from build123d import *

# Parameters (mm, degrees)
SKETCH1_W           = 41.35
SKETCH1_H           = 35
BOSS_EXTRUDE1_DEPTH = 3.175
SKETCH2_W           = 28.65
SKETCH2_H           = 7.5
SKETCH2_W_2         = 13.075
SKETCH2_H_2         = 3.175
SKETCH2_W_3         = 14.9
CUT_EXTRUDE1_DEPTH  = 4.175


with BuildPart() as part:
    # Sketch1 → Boss-Extrude1 (new body)
    with BuildSketch(Plane(origin=(0, 0, 0), x_dir=(1, 0, 0), z_dir=(0, 1, 0))):
        with Locations((20.675, 17.5)):
            Rectangle(SKETCH1_W, SKETCH1_H)
    extrude(amount=BOSS_EXTRUDE1_DEPTH)

    # Sketch2 → Cut-Extrude1 (cut, through all)
    with BuildSketch(Plane(origin=(0, 3.175, 0), x_dir=(1, 0, 0), z_dir=(0, 1, 0))):
        with Locations((20.675, 23.75)):
            Rectangle(SKETCH2_W, SKETCH2_H)
        with Locations((6.5375, 33.4125)):
            Rectangle(SKETCH2_W_2, SKETCH2_H_2)
        with Locations((34.8125, 33.4125)):
            Rectangle(SKETCH2_W_2, SKETCH2_H_2)
        Polygon((38.175, 21.825), (41.35, 21.825), (41.35, 11.15), (28.275, 11.15), (28.275, 14.325), (38.175, 14.325), align=None)
        Polygon((3.175, 21.825), (3.175, 14.325), (13.075, 14.325), (13.075, 11.15), (0, 11.15), (0, 21.825), align=None)
        with Locations((33.9, 1.5875)):
            Rectangle(SKETCH2_W_3, SKETCH2_H_2)
        with Locations((7.45, 1.5875)):
            Rectangle(SKETCH2_W_3, SKETCH2_H_2)
    extrude(amount=-CUT_EXTRUDE1_DEPTH, mode=Mode.SUBTRACT)


solid = part.part
Source: CAD feature listing. Evaluate the final solid. Frame: model axes, mm. A direction names the side the tool comes from. Round coordinates to 2 decimals unless told otherwise and drop trailing zeros. Loops run counter-clockwise (first coordinate to the right, second up) from the corner with the lowest first, then second, coordinate; pieces in that order, holes last.
Q1. First-contact query: P1, Ø1, axis at x = 40.5, y = 2.5, coming from the +Z side (3 decimals); P2, Ø1, axis at y = 1.5, z = -1.5, coming from the -X side; P3, Ø1, axis at y = 2, z = -33, coming from the -X side (3 decimals). Flat tips, straight axial feed; report the tip coordinate or a pass-through.
Q2. Access query for faces 5 (the face through (26.45, 2, -2)), 6 (the face through (40, 2, -21.825)), 7 (the face through (7, 2, -3.175)), 8 (the face through (7, 2, -11.15)). Directions: +Z, -Z, +X, -X, +Y, -Y. A direction counts if a zero-diameter tool reaches every point of the face in a straight line with its end or side. Return the directions, or none.
Q3. Ray query, line 1 (Z direction, x = 10, y = 2.45) (3 decimals); line 2 (Z direction, x = 27, y = 1.9) (3 decimals); line 3 (Z direction, x = 4.5, y = 2.7) (3 decimals). Return the intervals inside material, ascending.
Q4. Mould query, pull axis X, two halves, no side actions, for faces 1 (the face through (35, 2, -31.825)), 2 (the face through (3.175, 2, -18)), 3 (the face through (20, 2, -20)), 4 (the face through (6.35, 2, -24)). Classes: pulls with the +X half, pulls with the -X half, needs draft (parallel to the pull), parting line crosses it, or undercut.
Q5. Section D-D, the plane y = 1.95. Return loops of the section in (x, z) (3 decimals), plus the area to 3 significant figures.
Q6. Section A-A, the plane z = -23.5. Return loops of the section in (x, y) (3 decimals).
Q7. Section B-B, the plane x = 10. Return loops of the section in (y, z) (3 decimals), plus the area to 3 significant figures.
Q8. Section C-C, the plane x = 19. Return loops of the section in (y, z) (3 decimals).
Solutions:
1. P1: stops at z = -3.175
1. P2: stops at x = 14.9
1. P3: stops at x = 13.075
2. face 5: +Z, +X, +Y, -Y
2. face 6: +X, +Y, -Y
2. face 7: +Z, -X, +Y, -Y
2. face 8: -X, +Y, -Y
3. line 1: z = -31.825 to -27.5, -20 to -14.325, -11.15 to -3.175
3. line 2: z = -35 to -27.5, -20 to -3.175
3. line 3: z = -31.825 to -14.325, -11.15 to -3.175
4. face 1: needs draft
4. face 2: pulls with the -X half
4. face 3: undercut
4. face 4: undercut
5. outline: (0, -31.825) - (13.075, -31.825) - (13.075, -35) - (28.275, -35) - (28.275, -31.825) - (41.35, -31.825) - (41.35, -21.825) - (38.175, -21.825) - (38.175, -14.325) - (28.275, -14.325) - (28.275, -11.15) - (41.35, -11.15) - (41.35, -3.175) - (26.45, -3.175) - (26.45, 0) - (14.9, 0) - (14.9, -3.175) - (0, -3.175) - (0, -11.15) - (13.075, -11.15) - (13.075, -14.325) - (3.175, -14.325) - (3.175, -21.825) - (0, -21.825) - close; hole (6.35, -27.5) - (35, -27.5) - (35, -20) - (6.35, -20) - close
5. area: 924 mm2
6. outline: (0, 0) - (6.35, 0) - (6.35, 3.175) - (0, 3.175) - close; (35, 0) - (41.35, 0) - (41.35, 3.175) - (35, 3.175) - close
7. outline: (0, -31.825) - (3.175, -31.825) - (3.175, -27.5) - (0, -27.5) - close; (0, -20) - (3.175, -20) - (3.175, -14.325) - (0, -14.325) - close; (0, -11.15) - (3.175, -11.15) - (3.175, -3.175) - (0, -3.175) - close
7. area: 57.1 mm2
8. outline: (0, -35) - (3.175, -35) - (3.175, -27.5) - (0, -27.5) - close; (0, -20) - (3.175, -20) - (3.175, 0) - (0, 0) - close
